Geometry: final body of the model. Coordinates: model frame, mm. Face numbers are marked on the shaded views. Coordinates: 2 decimals unless noted, no trailing zeros. Order: outer loops, then holes, each group sorted by start corner. A loop starts at its lowest first (then second) coordinate and runs counter-clockwise, first axis right, second up. Notation, with made-up numbers: M 31.5,66 L 72.5,66 A16 ccw 72.5,88 Z; hole C 2.5,-31.75 d11. An arc over 180 degrees is marked long. Use CSV: the item, a comma, the result in double quotes. Start each with the question number.
1. Section query D-D on z = 22. Return the cut outline in (x, y), and give its area (3 significant figures).
2. Section query B-B on y = 0. Return the cut outline in (x, z), and give its area (3 significant figures).
3. First-contact query: P1, Ø1.5, axis at x = 8, z = 14.5, coming from the -Y side; P2, Ø5, axis at y = 3.5, z = 17, coming from the -X side; P3, Ø8, axis at x = -7.5, z = 16.5, coming from the -Y side. Flat tips, straight axial feed; report the tip coordinate or a pass-through.
4. Material intervals for line 1 (Y direction, x = 0, z = 3.25); line 2 (X direction, y = 0.75, z = 14.75); line 3 (X direction, y = -5.5, z = 20), sorted ascending.
5. Pull-direction query (Y, two-part tool) for the marked faces 1, 2, 3 and 4; classes: pulls with the +Y half, pulls with the -Y half, needs draft (parallel to the pull), parting line crosses it, or undercut.
6. Section query C-C on y = -6. Return the cut outline in (x, z), and give its area (3 significant figures).
7. Section query A-A on x = -0.75. Return the cut outline in (y, z).
from build123d import *

# Parameters (mm, degrees)
F0_R     = 10.16
F1_DEPTH = 25.4
F2_R     = 2.794
F3_DEPTH = 76.2
F4_R     = 6.35
F5_DEPTH = 12.7


with BuildPart() as f1:
    # F0 (on Top) → F1 (new body)
    with BuildSketch(Plane.XY):
        Circle(F0_R)
    extrude(amount=F1_DEPTH)

    # F2 (on face) → F3 (cut)
    with BuildSketch(Plane.XY):
        Circle(F2_R)
    extrude(amount=F3_DEPTH, mode=Mode.SUBTRACT)

    # F4 (on face) → F5 (cut)
    with BuildSketch(Plane.XY.offset(25.4)):
        Circle(F4_R)
    extrude(amount=-F5_DEPTH, mode=Mode.SUBTRACT)


solid = f1.part
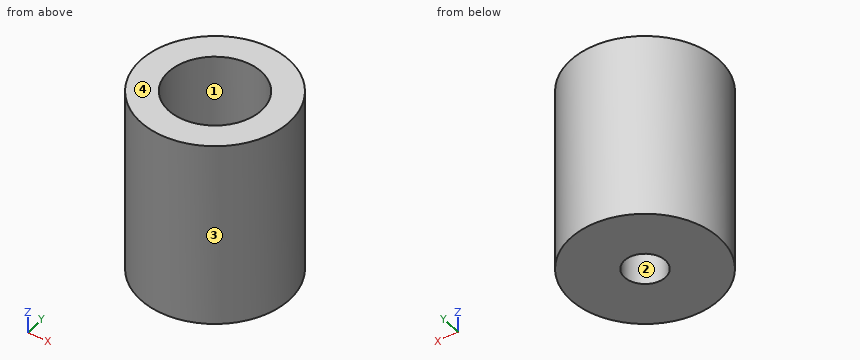
Results list:
1,outline,"C 0,0 d20.32; hole C 0,0 d12.7"
1,area,"198 mm²"
2,outline,"M -10.16,0 L -2.79,0 L -2.79,12.7 L -6.35,12.7 L -6.35,25.4 L -10.16,25.4 Z; M 2.79,0 L 10.16,0 L 10.16,25.4 L 6.35,25.4 L 6.35,12.7 L 2.79,12.7 Z"
2,area,"284 mm²"
3,P1,"stops at y = -7.12"
3,P2,"stops at x = -10.11"
3,P3,"stops at y = -9.54"
4,line 1,"y = -10.16 to -2.79, 2.79 to 10.16"
4,line 2,"x = -10.13 to -6.31, 6.31 to 10.13"
4,line 3,"x = -8.54 to -3.17, 3.17 to 8.54"
5,face 1,"undercut"
5,face 2,"undercut"
5,face 3,"parting line crosses it"
5,face 4,"needs draft"
6,outline,"M -8.2,0 L 8.2,0 L 8.2,25.4 L 2.08,25.4 L 2.08,12.7 L -2.08,12.7 L -2.08,25.4 L -8.2,25.4 Z"
6,area,"364 mm²"
7,outline,"M -10.13,0 L -2.69,0 L -2.69,12.7 L -6.31,12.7 L -6.31,25.4 L -10.13,25.4 Z; M 2.69,0 L 10.13,0 L 10.13,25.4 L 6.31,25.4 L 6.31,12.7 L 2.69,12.7 Z"
